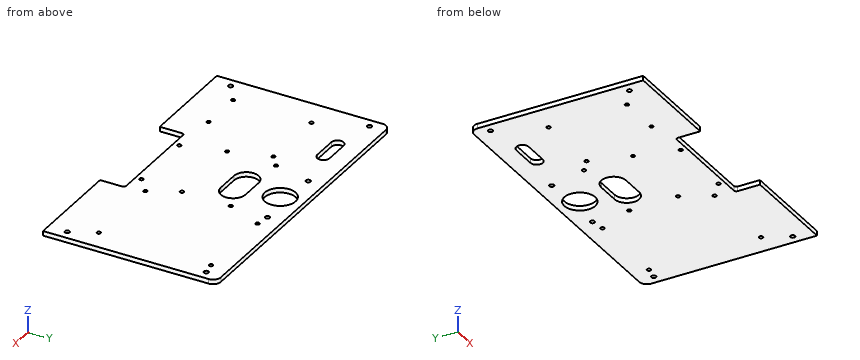
from build123d import *

# Parameters (mm, degrees)
SKETCH_W      = 198
SKETCH_H      = 112.5
PAD_DEPTH     = 3
FILLET_R      = 5
SKETCH001_R   = 1.5
SKETCH001_R_2 = 10
SKETCH001_R_3 = 1.25
POCKET_DEPTH  = 3.001


with BuildPart() as part:
    # Sketch → Pad (new body)
    with BuildSketch(Plane.XY):
        Rectangle(SKETCH_W, SKETCH_H)
    extrude(amount=PAD_DEPTH)

    # Fillet
    fillet_edges = [part.edges().sort_by_distance(p)[0] for p in [
        (-99, 56.25, 1.5),
        (99, 56.25, 1.5),
    ]]
    fillet(fillet_edges, radius=FILLET_R)

    # Sketch001 (on Face5 of Fillet) → Pocket (cut, through all)
    with BuildSketch(Plane.XY.offset(3)):
        with Locations((-93, 46.25)):
            Circle(SKETCH001_R)
        with Locations((-93, -43.92)):
            Circle(SKETCH001_R)
        with Locations((93, 46.25)):
            Circle(SKETCH001_R)
        with Locations((93, -43.92)):
            Circle(SKETCH001_R)
        with Locations((-23.15, 46.25)):
            Circle(SKETCH001_R)
        with Locations((23.15, 46.25)):
            Circle(SKETCH001_R)
        with Locations((0, 41.25)):
            Circle(SKETCH001_R_2)
        with Locations((-21.59, -36.5)):
            Circle(SKETCH001_R_3)
        with Locations((21.59, -36.5)):
            Circle(SKETCH001_R_3)
        with Locations((-29, 22)):
            Circle(SKETCH001_R_3)
        with Locations((-29, -9.75)):
            Circle(SKETCH001_R_3)
        with Locations((22.43, -9.75)):
            Circle(SKETCH001_R_3)
        with Locations((22.43, 22)):
            Circle(SKETCH001_R_3)
        with Locations((-80.18, 15.8)):
            Circle(SKETCH001_R_3)
        with Locations((-37, 15.8)):
            Circle(SKETCH001_R_3)
        with Locations((-80.18, -35)):
            Circle(SKETCH001_R_3)
        with Locations((32, 44.8)):
            Circle(SKETCH001_R_3)
        with Locations((85, 44.8)):
            Circle(SKETCH001_R_3)
        with Locations((32, -28)):
            Circle(SKETCH001_R_3)
        with Locations((85, -28)):
            Circle(SKETCH001_R_3)
        with Locations((-52.24, -35)):
            Circle(SKETCH001_R_3)
        with BuildLine():
            Line((-32.5, -40.25), (32.5, -40.25))
            ThreePointArc((34, -41.75), (33.56066, -40.68934), (32.5, -40.25))
            Line((34, -41.75), (34, -56.25))
            Line((34, -56.25), (-34, -56.25))
            Line((-34, -56.25), (-34, -41.75))
            ThreePointArc((-32.5, -40.25), (-33.56066, -40.68934), (-34, -41.75))
        make_face()
        with BuildLine():
            ThreePointArc((-67, 44.25), (-71, 40.25), (-67, 36.25))
            Line((-67, 36.25), (-51, 36.25))
            ThreePointArc((-51, 36.25), (-47, 40.25), (-51, 44.25))
            Line((-67, 44.25), (-51, 44.25))
        make_face()
        with BuildLine():
            ThreePointArc((-7.5, 23), (-15.5, 15), (-7.5, 7))
            Line((-7.5, 7), (7.5, 7))
            ThreePointArc((7.5, 7), (15.5, 15), (7.5, 23))
            Line((-7.5, 23), (7.5, 23))
        make_face()
    extrude(amount=-POCKET_DEPTH, mode=Mode.SUBTRACT)


solid = part.part
Input: part model. Units: mm. Frame: model coordinates. Give positions to 0.01 mm unless a question says otherwise; leave off trailing zeros. Order: outer loops, then holes, each group sorted by start corner. A loop starts at its lowest first (then second) coordinate and runs counter-clockwise, first axis right, second up.
Q1. Section B-B on y = 33.5. Output: boundary loops of the cut face in (x, z), and give its area (3 significant figures).
Checked values:
outline: (-99, 0) - (-6.32, 0) - (-6.32, 3) - (-99, 3) - close; (6.32, 0) - (99, 0) - (99, 3) - (6.32, 3) - close
area: 556 mm2
Q2. Ray query, probe 1 along Y at (x, z) = (32, 0.8); probe 2 along Y at (x, z) = (93, 1.7); probe 3 along Y at (x, z) = (-54.5, 0.2). Return the intervals inside material, ascending.
Checked values:
probe 1: y = -40.25 to -29.25, -26.75 to 43.55, 46.05 to 56.25
probe 2: y = -56.25 to -45.42, -42.42 to 44.75, 47.75 to 56.25
probe 3: y = -56.25 to 36.25, 44.25 to 56.25
Q3. Section A-A on x = -65. Output: boundary loops of the cut face in (y, z), and give its area (4 significant figures).
Checked values:
outline: (-56.25, 0) - (36.25, 0) - (36.25, 3) - (-56.25, 3) - close; (44.25, 0) - (56.25, 0) - (56.25, 3) - (44.25, 3) - close
area: 313.5 mm2
Q4. Section D-D on z = 0.5. State how many separate pieces and enclosed holes the cut face has, and give its area (3 significant figures).
Checked values:
separate pieces: 1
enclosed holes: 23
area: 20,100 mm2
Q5. Contact query for flat-ended pins moving along their axis: pin 1 Ø2 at (x, y) = (-21.59, -36.5) entering from +Z; pin 2 Ø0.9 at (x, z) = (-1, 2) entering from -Y. Output: stop coordinate, or through.
Checked values:
pin 1: passes through
pin 2: stops at y = -40.25
Q6. Section C-C on x = 5. Output: boundary loops of the cut face in (y, z), and give its area (3 significant figures).
Checked values:
outline: (-40.25, 0) - (7, 0) - (7, 3) - (-40.25, 3) - close; (23, 0) - (32.59, 0) - (32.59, 3) - (23, 3) - close; (49.91, 0) - (56.25, 0) - (56.25, 3) - (49.91, 3) - close
area: 190 mm2
